Verification items for the finished model (mm, model axes). A direction names the side the tool comes from. Coordinates: 2 decimals unless noted, no trailing zeros. Order: outer loops, then holes, each group sorted by start corner. A loop starts at its lowest first (then second) coordinate and runs counter-clockwise, first axis right, second up. Notation, with made-up numbers: M -33,21 L -6,21 A31 cw -6,52 Z; hole C -20.75,68.25 d3. An arc over 180 degrees is marked long. Return JSON: item names as keys, results as strings. Group by question number.
Q1. Thickness scan on probe 1 along Z at (x, y) = (-7.25, -8); probe 2 along X at (y, z) = (-0.25, 9); probe 3 along Y at (x, z) = (0, 9). Record the ranges inside material, lowest first.
Q2. Access from +Z, -Z, +X, -X, +Y, -Y to the whole of each face (thin tool, end or side, straight path). Record for faces 1 (the face through (3, 3, 19.05)), 2 (the face through (-1.38, -6.2, 0.16)), 3 (the face through (0, 2.877, 12)).
Q3. Go/stop test with flat-tipped pins: pin 1 Ø1.7 at (x, z) = (0.5, 12.5) entering from -Y; pin 2 Ø12 at (y, z) = (1, 2.5) entering from +X; pin 3 Ø10 at (x, z) = (-0.5, 4) entering from +Y; pin 4 Ø3 at (x, y) = (10, -7) entering from -Z. Record where each tip stops, or that it passes through.
Q4. Section check D-D, the plane z = -1. Enter the section's corners in (x, y), then the cut area to 3 significant figures.
Q5. Mould release check, pull along X, two halves, no side actions. Record for faces 4 (the face through (5.86, 11.267, 16.644)), 5 (the face through (-1, 9, 14.288)), 6 (the face through (0, 0, 5.08)): pulls with the +X half, pulls with the -X half, needs draft (parallel to the pull), parting line crosses it, or undercut.
from build123d import *

# Parameters (mm, degrees)
SKETCH1_R                = 6.35
SKETCH1_R_2              = 3.317499969
BOSS_EXTRUDE1_DEPTH      = 14.2875
BOSS_EXTRUDE1_DEPTH_BACK = 14.2875
SKETCH2_R                = 12.7
SKETCH2_R_2              = 6.35
SKETCH2_R_3              = 3.317499969
BOSS_EXTRUDE3_DEPTH      = 4.7625
SKETCH3_R                = 3.317499969
BOSS_EXTRUDE4_DEPTH      = 24.13
FILLET1_R                = 2.54
CHAMFER1_SIZE            = 0.635
BOSS_EXTRUDE5_REACH      = 44.121


with BuildPart() as part:
    # Sketch1 → Boss-Extrude1 (new, two sides)
    with BuildSketch(Plane.XY) as boss_extrude1_sk:
        Circle(SKETCH1_R)
        Circle(SKETCH1_R_2, mode=Mode.SUBTRACT)
    extrude(amount=BOSS_EXTRUDE1_DEPTH)
    extrude(boss_extrude1_sk.sketch, amount=-BOSS_EXTRUDE1_DEPTH_BACK)

    # Sketch2 → Boss-Extrude3 (add)
    with BuildSketch(Plane(origin=(0, 0, -14.2875), x_dir=(-1, 0, 0), z_dir=(0, 0, -1))):
        with Locations(Location((0, 0, 0), (0, 0, 180))):
            Circle(SKETCH2_R)
        with Locations(Location((0, 0, 0), (0, 0, 180))):
            Circle(SKETCH2_R_2, mode=Mode.SUBTRACT)
        with Locations(Location((0, 0, 0), (0, 0, 180))):
            Circle(SKETCH2_R_2)
        with Locations(Location((0, 0, 0), (0, 0, 180))):
            Circle(SKETCH2_R_3, mode=Mode.SUBTRACT)
    boss_extrude3 = extrude(amount=BOSS_EXTRUDE3_DEPTH)

    # Mirror1: Boss-Extrude3 across plane
    add(boss_extrude3.mirror(Plane.XY))

    # Sketch3 → Boss-Extrude4 (add)
    with BuildSketch(Plane(origin=(0, 0, -19.05), x_dir=(-1, 0, 0), z_dir=(0, 0, -1))):
        Circle(SKETCH3_R)
    extrude(amount=-BOSS_EXTRUDE4_DEPTH)

    # Fillet1
    fillet1_edges = [part.edges().sort_by_distance(p)[0] for p in [
        (-6.35, 0, -14.2875),
        (-6.35, 0, 14.2875),
    ]]
    fillet(fillet1_edges, radius=FILLET1_R)

    # Chamfer1
    chamfer1_edges = [part.edges().sort_by_distance(p)[0] for p in [
        (-12.7, 0, -14.2875),
        (-12.7, 0, -19.05),
        (-12.7, 0, 19.05),
        (-12.7, 0, 14.2875),
    ]]
    chamfer(chamfer1_edges, length=CHAMFER1_SIZE)

    # Sketch4 → Boss-Extrude5 (add, up to next)
    with BuildSketch(Plane.XY.offset(19.05), mode=Mode.PRIVATE) as boss_extrude5_sk1:
        with BuildLine():
            ThreePointArc((1.651, 2.87749979), (0, 3.317499969), (-1.651, 2.87749979))
            Line((-1.651, 2.87749979), (1.651, 2.87749979))
        make_face()
    boss_extrude5_tool1 = extrude(boss_extrude5_sk1.sketch, amount=-BOSS_EXTRUDE5_REACH, mode=Mode.PRIVATE) - part.part
    add(boss_extrude5_tool1.solids().sort_by_distance((0, 3.05454, 19.05))[0])


solid = part.part
Numbers:
{
 "1": {"probe 1": "z = -19.05 to -14.29, 14.29 to 19.05", "probe 2": "x = -6.35 to -3.31, 3.31 to 6.35", "probe 3": "y = -6.35 to -3.32, 2.88 to 6.35"},
 "2": {"face 1": "+Z, +X, -X, +Y, -Y", "face 2": "none", "face 3": "+Z"},
 "3": {"pin 1": "stops at y = -6.9", "pin 2": "stops at x = 6.35", "pin 3": "stops at y = 6.35", "pin 4": "stops at z = -19.05"},
 "4": {"outline": "C 0,0 d12.7", "area": "127 mm2"},
 "5": {"face 4": "parting line crosses it", "face 5": "needs draft", "face 6": "undercut"}
}
